CAD build for the part. Positions are in the model's coordinates, mm. A direction names the side the tool comes from. Coordinates: 2 decimals unless noted, no trailing zeros. Loops run counter-clockwise (first coordinate to the right, second up) from the corner with the lowest first, then second, coordinate; pieces in that order, holes last. Notation, with made-up numbers: (81.25, 0.25) -> (102.25, 0.25) arc R24 cw to (102.25, 32.25) -> close; hole circle Ø10 at (-20.75, -2). An arc over 180 degrees is marked (long way). Write each question's results on one line, items separated by ' | '.
Autodesk Inventor part; units mm, degrees
ref_plane "YZ Plane" through (0, 0, 0) normal (1, 0, 0) x (0, 1, 0)
ref_plane "XZ Plane" through (0, 0, 0) normal (0, 1, 0) x (-1, 0, 0)
ref_plane "XY Plane" through (0, 0, 0) normal (0, 0, 1) x (1, 0, 0)
sketch "Skizze1" plane through (0, 0, 0) normal (0, 0, 1) x (1, 0, 0)
  line L0 (-10.271, 0) -> (24.729, 0)
  line L1 (0, -27.3364) -> (0, 7.6636)
  line L2 (16.729, -0.3364) -> (-5.271, -0.3364)
  line L3 (-5.271, -0.3364) -> (-5.271, 2.6636)
  line L4 (-5.271, 2.6636) -> (19.729, 2.6636)
  line L5 (19.729, 2.6636) -> (19.729, -22.3364)
  line L6 (19.729, -22.3364) -> (16.729, -22.3364)
  line L7 (16.729, -0.3364) -> (16.729, -22.3364)
  point P0 (0, 0)
  dimension "d0" = 3
  dimension "d1" = 3
  dimension "d2" = 25
  dimension "d3" = 25
extrude "Extrusion1" add sketch "Skizze1" along normal blind 100
sketch "Skizze2" plane through (19.729, -22.3364, 0) normal (1, 0, 0) x (0, 0, -1)
  line L0 (0, 25) -> (-100, 25)
  line L1 (-100, 0) -> (-100, 25)
  line L2 (0, 0) -> (0, 25)
  point P0 (0, 22.3364)
  point P1 (-91.5, 12.5)
  point P2 (-8.5, 12.5)
  dimension "d6" = 12.5
  dimension "d7" = 12.5
  dimension "d8" = 8.5
  dimension "d9" = 8.5
hole "Bohrung1" at (19.729, -9.8364, 91.5) at (19.729, -9.8364, 8.5) direction (-1, 0, 0) diameter 2.459 depth 8.8 tip angle 118
properties part number "Halter vorne"
1) Slice it at A-A (z = 91.5). Write the cut outline in (x, y), then the cut area to 3 significant figures.
Outcome:
outline: (-5.27, -0.34) -> (16.73, -0.34) -> (16.73, -8.61) -> (19.73, -8.61) -> (19.73, 2.66) -> (-5.27, 2.66) -> close; (16.73, -22.34) -> (19.73, -22.34) -> (19.73, -11.07) -> (16.73, -11.07) -> close | area: 134 mm^2
2) Slice it at B-B (z = 41.5). Write the cut outline in (x, y).
Outcome:
outline: (-5.27, -0.34) -> (16.73, -0.34) -> (16.73, -22.34) -> (19.73, -22.34) -> (19.73, 2.66) -> (-5.27, 2.66) -> close
3) Pin check, flat tips, straight feed: pin 1 (1 mm diameter, centred on x = 0, z = 33, fed in from -Y); pin 2 (8 mm diameter, centred on y = -9, z = 48, fed in from -X). Stop position of each tip, or through.
Outcome:
pin 1: stops at y = -0.34 | pin 2: stops at x = 16.73
4) Which spindle directions (+Z, -Z, +X, -X, +Y, -Y) get a long thin tool onto all of the face, cutting with end or side? Do faces 1 (the flat face through (16.729, -11, 49)), 2 (the flat face through (-5.271, 1, 49)). Say none if no direction does.
Outcome:
face 1: +Z, -Z, -X, -Y | face 2: +Z, -Z, -X, +Y, -Y
5) Slice it at C-C (x = 9.75). Write the cut outline in (y, z), then the cut area to 3 significant figures.
Outcome:
outline: (-0.34, 0) -> (2.66, 0) -> (2.66, 100) -> (-0.34, 100) -> close | area: 300 mm^2
6) Two-plate mould, pull along Z, no slides. Class faces 3 (the cylindrical face through (18.208, -8.746, 7.933)), 4 (the flat face through (12, 0, 100)), 5 (the flat face through (6, -0.336, 49)): pulls with the +Z half, pulls with the -Z half, needs draft (parallel to the pull), parting line crosses it, or undercut.
Outcome:
face 3: undercut | face 4: pulls with the +Z half | face 5: needs draft
7) Drill centre lines: L1, parallel to Y at x = 18, z = 91.5; L2, parallel to X at y = -17.5, z = 69; L3, parallel to Y at x = 10.75, z = 13.5. Where is each one in solid material? Low to high. Write a range as from..to.
Outcome:
L1: y = -22.34..-11.07, -8.61..2.66 | L2: x = 16.73..19.73 | L3: y = -0.34..2.66
